Here's how the part is built. I have some questions about the finished solid (model axes, mm). A direction names the side the tool comes from. Coordinates: 2 decimals unless noted, no trailing zeros. Order: outer loops, then holes, each group sorted by start corner. A loop starts at its lowest first (then second) coordinate and runs counter-clockwise, first axis right, second up. Notation, with made-up numbers: M 74.25,86.5 L 78.25,86.5 A23 cw 78.25,109.5 Z; hole C 19,13.5 d6. An arc over 180 degrees is marked long. Answer as CSV lines item,"result". Start each with the question number.
```python
from build123d import *

# Parameters (mm, degrees)
F0_W     = 450
F0_H     = 450
F1_DEPTH = 950
F2_W     = 50
F2_H     = 50
F2_W_2   = 330
F2_H_2   = 425
F3_DEPTH = 450.001
F4_W     = 380
F4_H     = 425
F5_DEPTH = 450.001


with BuildPart() as f1:
    # F0 (on Top) → F1 (new body)
    with BuildSketch(Plane.XY):
        Rectangle(F0_W, F0_H)
    extrude(amount=F1_DEPTH)

    # F2 (on face) → F3 (cut, through all)
    with BuildSketch(Plane.YZ.offset(225)):
        with Locations((200, 450)):
            Rectangle(F2_W, F2_H)
        Polygon((-225, 950), (-225, 475), (140, 475), (190, 950), align=None)
        Polygon((225, 950), (175, 475), (225, 475), align=None)
        with Locations((-25, 212.5)):
            Rectangle(F2_W_2, F2_H_2)
        with Locations((200, 212.5)):
            Rectangle(F2_W, F2_H_2)
    extrude(amount=-F3_DEPTH, mode=Mode.SUBTRACT)

    # F4 (on face) → F5 (cut, through all)
    with BuildSketch(Plane.XZ.offset(225)):
        with Locations((0, 212.5)):
            Rectangle(F4_W, F4_H)
    extrude(amount=-F5_DEPTH, mode=Mode.SUBTRACT)


solid = f1.part
```
1) Suppose I cut it at D-D on z = 726. Please give me the cut outline in (x, y), plus the area to 4 significant figures.
2) Which directions (+Z, -Z, +X, -X, +Y, -Y) give clear straight access to the entire face, cutting with the end or side of a thin tool? Please do faces 1 (the face through (-190, -208, 210)), 2 (the face through (1, 175, 432)), 3 (the face through (-207, 140, 210)), 4 (the face through (3, -45, 475)).
3) Suppose I cut it at C-C on y = -69.5. Please give me the cut outline in (x, z).
4) Suppose I cut it at A-A on z = 206. Please give me the cut outline in (x, y), plus the area to 3 significant figures.
5) If we mould it in two halves opening along Y, with no side actions, what happens to faces 5 (the face through (-207, -190, 210)), 6 (the face through (208, 140, 210)), 7 (the face through (3.15, 200.35, 715.82)), 8 (the face through (190, 157, 210))? For each: released by +Y, released by -Y, zero draft, split by the parting line, or undercut.
6) I need wall thicknesses on line 1 (X direction, y = -199, z = 384); line 2 (Z direction, x = 39.5, y = -87.5); line 3 (Y direction, x = 97, z = 670). Which ranges of each line are inside material? Lowest first, please. Write a range as [from, to].
7) Will these pins go through, and if not, where does the flat tip stop? pin 1 Ø2 at (x, y) = (-135, 27.5) entering from +Z; pin 2 Ø1 at (x, z) = (25, 491) entering from +Y; pin 3 Ø10.5 at (x, z) = (-208, 218.5) entering from +Y.
8) Suppose I cut it at B-B on x = -104.5. Please give me the cut outline in (y, z).
Output:
1,outline,"M -225,166.42 L 225,166.42 L 225,201.42 L -225,201.42 Z"
1,area,"15,750 mm²"
2,face 1,"-Z, +Y, -Y"
2,face 2,"-Z, +X, -X, +Y"
2,face 3,"-Z, +X, -X"
2,face 4,"+Z, +X, -X, -Y"
3,outline,"M -225,425 L 225,425 L 225,475 L -225,475 Z"
4,outline,"M -225,-225 L -190,-225 L -190,-190 L -225,-190 Z; M -225,140 L -190,140 L -190,175 L -225,175 Z; M 190,-225 L 225,-225 L 225,-190 L 190,-190 Z; M 190,140 L 225,140 L 225,175 L 190,175 Z"
4,area,"4,900 mm²"
5,face 5,"undercut"
5,face 6,"undercut"
5,face 7,"released by +Y"
5,face 8,"zero draft"
6,line 1,"[-225, -190], [190, 225]"
6,line 2,"[425, 475]"
6,line 3,"[160.53, 195.53]"
7,pin 1,"z = 475"
7,pin 2,"y = 176.74"
7,pin 3,"y = 175"
8,outline,"M -225,425 L 175,425 L 175,475 L 225,950 L 190,950 L 140,475 L -225,475 Z"
